```python
from build123d import *

# Parameters (mm, degrees)
SKETCH1_R                = 34.458333333
SKETCH1_R_2              = 3
BOSS_EXTRUDE1_DEPTH      = 5.7
CUT_EXTRUDE2_DEPTH       = 50.063667537
FILLET1_R                = 5.08
FILLET2_R                = 1.27
SKETCH2_R                = 0.79375
CUT_EXTRUDE1_DEPTH       = 50.063667537
M3_CLEARANCE_HOLE2_D     = 3.2
M3_CLEARANCE_HOLE2_DEPTH = 12.7
M3_CLEARANCE_HOLE2_TIP   = 0.96137699


with BuildPart() as part:
    # Sketch1 → Boss-Extrude1 (new body)
    with BuildSketch(Plane.XY):
        Circle(SKETCH1_R)
        Circle(SKETCH1_R_2, mode=Mode.SUBTRACT)
    extrude(amount=BOSS_EXTRUDE1_DEPTH)

    # Sketch3 → Cut-Extrude2 (cut, through all)
    with BuildSketch(Plane.XY.offset(5.7)):
        with BuildLine():
            Line((-3.652101058, 11.175), (-32.595952373, 11.175))
            ThreePointArc((-32.595952373, 11.175), (-31.293969256, 14.424431508), (-29.669026123, 17.525))
            Line((-29.669026123, 17.525), (-16.969026123, 17.525))
            Line((-16.969026123, 17.525), (-16.969026123, 20.7))
            Line((-16.969026123, 20.7), (-3.652101058, 20.7))
            Line((-3.652101058, 20.7), (-3.652101058, 23.875))
            Line((-3.652101058, 23.875), (2.147898942, 23.875))
            Line((2.147898942, 23.875), (2.147898942, 20.7))
            Line((2.147898942, 20.7), (21.197898942, 20.7))
            Line((21.197898942, 20.7), (21.197898942, 11.175))
            Line((21.197898942, 11.175), (2.147898942, 11.175))
            Line((2.147898942, 11.175), (2.147898942, 8))
            Line((2.147898942, 8), (-3.652101058, 8))
            Line((-3.652101058, 8), (-3.652101058, 11.175))
        make_face()
    extrude(amount=-CUT_EXTRUDE2_DEPTH, mode=Mode.SUBTRACT)

    # Fillet1
    fillet1_edges = [part.edges().sort_by_distance(p)[0] for p in [
        (-32.595952373, 11.175, 2.85),
    ]]
    fillet(fillet1_edges, radius=FILLET1_R)

    # Fillet2
    fillet2_edges = [part.edges().sort_by_distance(p)[0] for p in [
        (-29.669026123, 17.525, 2.85),
    ]]
    fillet(fillet2_edges, radius=FILLET2_R)

    # Sketch2 → Cut-Extrude1 (cut, through all)
    with BuildSketch(Plane.XY.offset(5.7)):
        with Locations((0, 12)):
            Circle(SKETCH2_R)
        with Locations((12, 0)):
            Circle(SKETCH2_R)
        with Locations((0, -12)):
            Circle(SKETCH2_R)
        with Locations((-12, 0)):
            Circle(SKETCH2_R)
        with Locations((-18, 26)):
            Circle(SKETCH2_R)
        with Locations((26, 18)):
            Circle(SKETCH2_R)
        with Locations((18, -26)):
            Circle(SKETCH2_R)
        with Locations((-26, -18)):
            Circle(SKETCH2_R)
    extrude(amount=-CUT_EXTRUDE1_DEPTH, mode=Mode.SUBTRACT)

    # M3 Clearance Hole2
    with Locations(Plane.XY.offset(5.7)):
        with Locations((-6, 0), (6, 0)):
            Hole(M3_CLEARANCE_HOLE2_D / 2, depth=M3_CLEARANCE_HOLE2_DEPTH)
            with Locations((0, 0, -(M3_CLEARANCE_HOLE2_DEPTH + M3_CLEARANCE_HOLE2_TIP / 2))):  # 118° drill point
                Cone(0, M3_CLEARANCE_HOLE2_D / 2, M3_CLEARANCE_HOLE2_TIP, mode=Mode.SUBTRACT)


solid = part.part
```
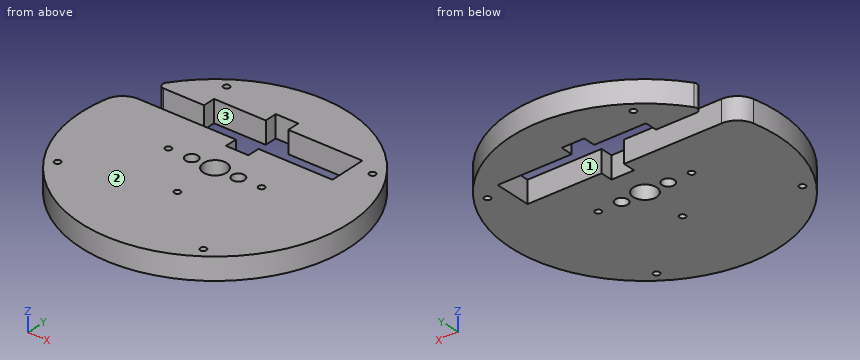
Verification items for the finished model (mm, model axes). Face numbers are marked on the shaded views. A direction names the side the tool comes from. Coordinates: 2 decimals unless noted, no trailing zeros. Order: outer loops, then holes, each group sorted by start corner. A loop starts at its lowest first (then second) coordinate and runs counter-clockwise, first axis right, second up. Notation, with made-up numbers: (48, -15.5) - (92, -15.5) arc R26 cw to (92, 8.5) - close; hole circle Ø6 at (65.25, 62). An arc over 180 degrees is marked (long way). Return JSON: item names as keys, results as strings.
(1) Section check A-A, the plane y = 0. Record the cut outline in (x, z), and give its area (3 significant figures).
Filled sheet:
{"outline": "(-34.46, 0) - (-12.79, 0) - (-12.79, 5.7) - (-34.46, 5.7) - close; (-11.21, 0) - (-7.6, 0) - (-7.6, 5.7) - (-11.21, 5.7) - close; (-4.4, 0) - (-3, 0) - (-3, 5.7) - (-4.4, 5.7) - close; (3, 0) - (4.4, 0) - (4.4, 5.7) - (3, 5.7) - close; (7.6, 0) - (11.21, 0) - (11.21, 5.7) - (7.6, 5.7) - close; (12.79, 0) - (34.46, 0) - (34.46, 5.7) - (12.79, 5.7) - close", "area": "304 mm^2"}
(2) Thickness scan on line 1 along Y through (x, z) = (0, 2.7) (3 decimals); line 2 along Y through (x, z) = (-18.5, 3.1) (3 decimals); line 3 along Y through (x, z) = (-2, 2.2) (3 decimals). Record the ranges inside material, lowest first.
Filled sheet:
{"line 1": "y = -34.458 to -12.794, -11.206 to -3, 3 to 8, 23.875 to 34.458", "line 2": "y = -29.071 to 11.175, 17.525 to 25.384, 26.616 to 29.071", "line 3": "y = -34.4 to -2.236, 2.236 to 8, 23.875 to 34.4"}
(3) Section check D-D, the plane x = -26. Record the cut outline in (y, z) (3 decimals), and give its area (3 significant figures).
Filled sheet:
{"outline": "(-22.614, 0) - (-18.794, 0) - (-18.794, 5.7) - (-22.614, 5.7) - close; (-17.206, 0) - (11.175, 0) - (11.175, 5.7) - (-17.206, 5.7) - close; (17.525, 0) - (22.614, 0) - (22.614, 5.7) - (17.525, 5.7) - close", "area": "213 mm^2"}
(4) Section check B-B, the plane x = 0. Record the cut outline in (y, z) (3 decimals).
Filled sheet:
{"outline": "(-34.458, 0) - (-12.794, 0) - (-12.794, 5.7) - (-34.458, 5.7) - close; (-11.206, 0) - (-3, 0) - (-3, 5.7) - (-11.206, 5.7) - close; (3, 0) - (8, 0) - (8, 5.7) - (3, 5.7) - close; (23.875, 0) - (34.458, 0) - (34.458, 5.7) - (23.875, 5.7) - close"}
(5) Go/stop test with flat-tipped pins: pin 1 (2 mm diameter, centred on x = 0, z = 4, fed in from +Y); pin 2 (2.5 mm diameter, centred on y = 23, z = 2, fed in from -X); pin 3 (3 mm diameter, centred on y = 27, z = 5, fed in from +X); pin 4 (9.5 mm diameter, centred on x = 0, y = 0, fed in from +Z). Record where each tip stops, or that it passes through.
Filled sheet:
{"pin 1": "stops at y = 34.46", "pin 2": "stops at x = -26.73", "pin 3": "stops at x = 23.18", "pin 4": "stops at z = 5.7"}
(6) Section check C-C, the plane y = -12. Record the cut outline in (x, z), and give its area (3 significant figures).
Filled sheet:
{"outline": "(-32.3, 0) - (-0.79, 0) - (-0.79, 5.7) - (-32.3, 5.7) - close; (0.79, 0) - (32.3, 0) - (32.3, 5.7) - (0.79, 5.7) - close", "area": "359 mm^2"}
(7) Access from +Z, -Z, +X, -X, +Y, -Y to the whole of each face (thin tool, end or side, straight path). Record for the marked faces 1, 2 and 3.
Filled sheet:
{"face 1": "+Z, -Z, -X", "face 2": "+Z, +X, -X, +Y, -Y", "face 3": "+Z, -Z"}
